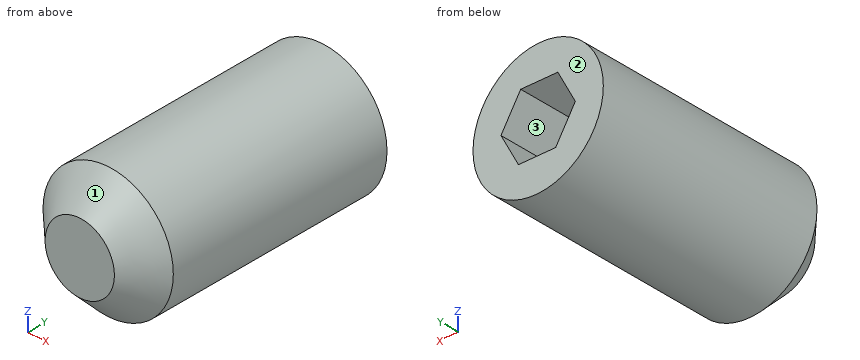
```python
from build123d import *

# Parameters (mm, degrees)
F0_R     = 2.3876
F1_DEPTH = 9.525
F3_DEPTH = 4.064
F4_SIZE  = 1.1176


with BuildPart() as f1:
    # F0 (on Front) → F1 (new body)
    with BuildSketch(Plane.XZ):
        Circle(F0_R)
    extrude(amount=-F1_DEPTH)

    # F2 (on face) → F3 (cut)
    with BuildSketch(Plane(origin=(0, 9.525, 0), x_dir=(-1, 0, 0), z_dir=(0, 1, 0))):
        Polygon((-1.363001, 0.047171), (-0.722352, -1.156808), (0.640649, -1.203979), (1.363001, -0.047171), (0.722352, 1.156808), (-0.640649, 1.203979), align=None)
    extrude(amount=-F3_DEPTH, mode=Mode.SUBTRACT)

    # F4
    f4_edges = [f1.edges().sort_by_distance(p)[0] for p in [
        (-2.3876, 0, 0),
    ]]
    chamfer(f4_edges, length=F4_SIZE)


solid = f1.part
```
Input: part model. Units: mm. Frame: model coordinates. Face numbers are marked on the shaded views. Coordinates: 2 decimals unless noted, no trailing zeros. Loops run counter-clockwise (first coordinate to the right, second up) from the corner with the lowest first, then second, coordinate; pieces in that order, holes last.
Q1. Section B-B, the plane x = 0. Return the cut outline in (y, z) (3 decimals), and give its area (3 significant figures).
Results are:
outline: (0, -1.27) - (1.118, -2.388) - (9.525, -2.388) - (9.525, -1.182) - (5.461, -1.182) - (5.461, 1.182) - (9.525, 1.182) - (9.525, 2.388) - (1.118, 2.388) - (0, 1.27) - close
area: 34.6 mm2
Q2. Section A-A, the plane y = 9. Return the cut outline in (x, z), and give its area (3 significant figures).
Results are:
outline: circle Ø4.78 at (0, 0); hole (-1.36, -0.05) - (-0.64, -1.2) - (0.72, -1.16) - (1.36, 0.05) - (0.64, 1.2) - (-0.72, 1.16) - close
area: 13.1 mm2
Q3. Section C-C, the plane y = 3.25. Return the cut outline in (x, z).
Results are:
outline: circle Ø4.78 at (0, 0)
Q4. Mould query, pull axis Z, two halves, no side actions, for the marked faces 1, 2 and 3. Classes: +Z half, -Z half, draft (parallel to the pull), parting line (faces both ways), or undercut.
Results are:
face 1: parting line
face 2: draft
face 3: undercut
Q5. Section D-D, the plane y = 1. Return the cut outline in (x, z), and give its area (3 significant figures).
Results are:
outline: circle Ø4.54 at (0, 0)
area: 16.2 mm2
Q6. Line query: line 1 along Z through (x, y) = (0.5, 6.5); line 2 along Z through (x, y) = (-1.25, 8.75); line 3 along X through (y, z) = (6, -0.65). Output: solid intervals per line, ascending.
Results are:
line 1: z = -2.33 to -1.16, 1.2 to 2.33
line 2: z = -2.03 to -0.23, 0.17 to 2.03
line 3: x = -2.3 to -0.99, 0.99 to 2.3
